Design review of the part built by this model. Coordinates are the model's own, in mm. A direction names the side the tool comes from. Round coordinates to 2 decimals unless told otherwise and drop trailing zeros. Loops run counter-clockwise (first coordinate to the right, second up) from the corner with the lowest first, then second, coordinate; pieces in that order, holes last. Notation, with made-up numbers: M 32.25,10 L 41.25,10 A29 cw 41.25,32 Z; hole C 51,49 d4. An arc over 180 degrees is marked long. One line per item, written item: value. Start each with the question number.
Item 1: We need section C-C (x = 19.75). Write out the cut boundary in (y, z), then the cut area to 3 significant figures.
Item 2: Mouldability with a two-part tool opening along Z and no side actions: class faces 4 (the cylindrical face through (8.427, 50.498, -69.865)), 5 (the cylindrical face through (31, 26.13, -77.07)), 6 (the cylindrical face through (8.427, 27.922, -86.435)) as released by +Z, released by -Z, zero draft, split by the parting line, or undercut.
Item 3: We need section D-D (z = -19). Write out the cut boundary in (x, y) (3 decimals), then the cut area to 3 significant figures.
Item 4: We need section A-A (y = 0). Write out the cut boundary in (x, z) (3 decimals), then the cut area to 3 significant figures.
Item 5: We need section B-B (z = -29). Write out the cut boundary in (x, y) (3 decimals).
Item 6: For faces 1 (the cylindrical face through (15.554, 0.185, -20.271)), 2 (the flat face through (8, 0, -72.769)), 3 (the flat face through (20, 28, -22)), list the 3-axis set-ups (+Z, -Z, +X, -X, +Y, -Y) from which the entire face can be reached by the end or side of a thin tool; tool diameter is ignored.
Item 7: Clearance check with flat-ended pins moving along their axes: pin 1 (4 mm diameter, centred on x = 19.5, z = -28, fed in from +Y); pin 2 (10 mm diameter, centred on x = 15.5, z = -65.5, fed in from +Y); pin 3 (8 mm diameter, centred on x = 23, y = 36.5, fed in from +Z); pin 4 (3.5 mm diameter, centred on x = 16, z = -82.5, fed in from +Y). State where each tip first meets the part, or that it passes through.
Item 8: For line 1 along Z through (x, y) = (20.25, -7.5); line 2 along Z through (x, y) = (7.25, 8); line 3 along Y through (x, z) = (19.75, -18.25), list the stretches that pass through material, from the lowest coordinate up.
from build123d import *

# Parameters (mm, degrees)
SKETCH1_R               = 4
BOSS_EXTRUDE1_DEPTH     = 39.5
CUT_EXTRUDE1_DEPTH      = 105.5
CUT_EXTRUDE1_DEPTH_BACK = 117.5
SKETCH2_W               = 25
SKETCH2_H               = 75.25
CUT_EXTRUDE2_DEPTH      = 43.5
SKETCH4_R               = 6
CUT_EXTRUDE3_DEPTH      = 41
SCALE1_SCALE            = 0.7


with BuildPart() as part:
    # Sketch1 → Boss-Extrude1 (new body)
    with BuildSketch(Plane(origin=(0, 0, 0), x_dir=(0, 0, -1), z_dir=(1, 0, 0))):
        with BuildLine():
            Line((0, -40), (0, 40))
            Line((0, 40), (25, 40))
            Line((25, 40), (73.280107592, 70.785366831))
            ThreePointArc((73.280107592, 70.785366831), (80.81695996, 72.117470486), (87.088258906, 67.730050596))
            Line((87.088258906, 67.730050596), (103.222887942, 42.426417539))
            ThreePointArc((103.222887942, 42.426417539), (104.391084837, 39.850237691), (104.791154167, 37.05))
            Line((104.791154167, 37.05), (104.791154167, -37.05))
            ThreePointArc((104.791154167, -37.05), (104.391084837, -39.850237691), (103.222887942, -42.426417539))
            Line((103.222887942, -42.426417539), (87.088258906, -67.730050596))
            ThreePointArc((87.088258906, -67.730050596), (80.81695996, -72.117470486), (73.280107592, -70.785366831))
            Line((73.280107592, -70.785366831), (25, -40))
            Line((25, -40), (0, -40))
        make_face()
        with Locations((78.7, 62.25)):
            Circle(SKETCH1_R, mode=Mode.SUBTRACT)
        with Locations((95, 37.153633057)):
            Circle(SKETCH1_R, mode=Mode.SUBTRACT)
        with Locations(Location((95, -37.153633057, 0), (0, 0, 180))):
            Circle(SKETCH1_R, mode=Mode.SUBTRACT)
        with Locations(Location((78.7, -62.25, 0), (0, 0, 180))):
            Circle(SKETCH1_R, mode=Mode.SUBTRACT)
        Polygon((30.81, -20), (30.81, 20), (75.651092334, 48.552793879), (84.857166207, 34.095), (84.857166207, -34.095), (75.651092334, -48.552793879), align=None, mode=Mode.SUBTRACT)
    extrude(amount=BOSS_EXTRUDE1_DEPTH)

    # Sketch2 → Cut-Extrude1 (cut, two sides: drawn at the far end of the back side and taken through both)
    with BuildSketch(Plane(origin=(0, 0, 0), x_dir=(1, 0, 0), z_dir=(0, 1, 0)).offset(-CUT_EXTRUDE1_DEPTH_BACK)):
        with Locations((19.75, 57.625)):
            Rectangle(SKETCH2_W, SKETCH2_H)
    extrude(amount=CUT_EXTRUDE1_DEPTH + CUT_EXTRUDE1_DEPTH_BACK, mode=Mode.SUBTRACT)

    # Sketch3 → Cut-Extrude2 (cut)
    with BuildSketch(Plane(origin=(0, 0, -104.791154167), x_dir=(-1, 0, 0), z_dir=(0, 0, -1))):
        Polygon((-7.25, -37.05), (-7.25, -12.5), (-32.25, -12.5), (-32.25, -37.05), (-32.25, -54.930146657), (-7.25, -54.930146657), align=None)
        Polygon((-32.25, 37.05), (-32.25, 12.5), (-7.25, 12.5), (-7.25, 37.05), (-7.25, 54.930146657), (-32.25, 54.930146657), align=None)
    extrude(amount=-CUT_EXTRUDE2_DEPTH, mode=Mode.SUBTRACT)

    # Sketch4 → Cut-Extrude3 (cut)
    with BuildSketch(Plane.XY):
        with Locations((19.75, 0)):
            Circle(SKETCH4_R)
    extrude(amount=-CUT_EXTRUDE3_DEPTH, mode=Mode.SUBTRACT)


with BuildPart() as part_1:
    # Scale1: scaled about (19.75, 0, -44.562080974)
    add(part.part.scale(SCALE1_SCALE).moved(Location((5.925, 0, -13.368624292))))


solid = part_1.part
A:
1. outline: M -28,-27.37 L -4.2,-27.37 L -4.2,-13.37 L -28,-13.37 Z; M -8.75,-86.72 L 8.75,-86.72 L 8.75,-80.04 L -8.75,-80.04 Z; M 4.2,-27.37 L 28,-27.37 L 28,-13.37 L 4.2,-13.37 Z
1. area: 783 mm2
2. face 4: split by the parting line
2. face 5: undercut
2. face 6: released by -Z
3. outline: M 5.925,-28 L 33.575,-28 L 33.575,28 L 5.925,28 Z; hole C 19.75,0 d8.4
3. area: 1,490 mm2
4. outline: M 5.925,-86.722 L 33.575,-86.722 L 33.575,-72.769 L 28.5,-72.769 L 28.5,-80.044 L 11,-80.044 L 11,-72.769 L 5.925,-72.769 Z; M 5.925,-34.936 L 11,-34.936 L 11,-27.369 L 15.55,-27.369 L 15.55,-13.369 L 5.925,-13.369 Z; M 23.95,-27.369 L 28.5,-27.369 L 28.5,-34.936 L 33.575,-34.936 L 33.575,-13.369 L 23.95,-13.369 Z
4. area: 605 mm2
5. outline: M 5.925,-28 L 11,-28 L 11,28 L 5.925,28 Z; M 28.5,-28 L 33.575,-28 L 33.575,28 L 28.5,28 Z
6. face 1: +Z
6. face 2: +X, -X
6. face 3: +Z, +X, -X, +Y
7. pin 1: y = 28
7. pin 2: y = 50.61
7. pin 3: through
7. pin 4: y = 8.75
8. line 1: -86.72 to -80.04, -27.37 to -13.37
8. line 2: -86.72 to -72.77, -34.94 to -13.37
8. line 3: -28 to -4.2, 4.2 to 28
